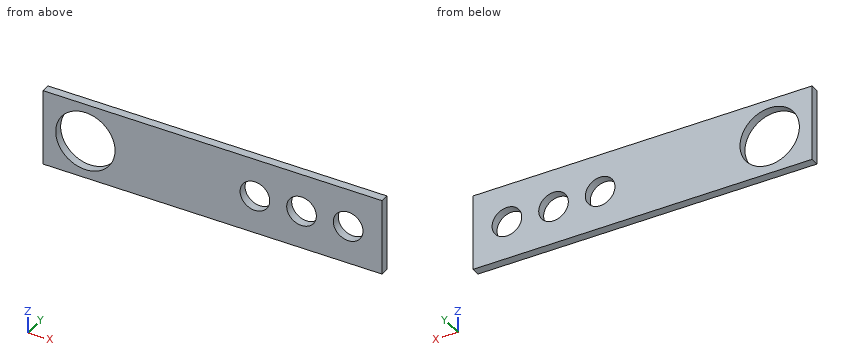
```python
from build123d import *

# Parameters (mm, degrees)
SKETCH2_W           = 40
SKETCH2_H           = 9
BOSS_EXTRUDE1_DEPTH = 1
SKETCH3_R           = 3.5
CUT_EXTRUDE1_DEPTH  = 3
SKETCH4_R           = 1.75
CUT_EXTRUDE2_DEPTH  = 3
LPATTERN1_COUNT     = 3
LPATTERN1_PITCH     = 5.5


with BuildPart() as part:
    # Sketch2 → Boss-Extrude1 (new body)
    with BuildSketch(Plane(origin=(0, 0, 0), x_dir=(1, 0, 0), z_dir=(0, 1, 0))):
        Rectangle(SKETCH2_W, SKETCH2_H)
    extrude(amount=BOSS_EXTRUDE1_DEPTH)

    # Sketch3 → Cut-Extrude1 (cut)
    with BuildSketch(Plane(origin=(0, 1, 0), x_dir=(1, 0, 0), z_dir=(0, 1, 0))):
        with Locations((-15, 0)):
            Circle(SKETCH3_R)
    extrude(amount=-CUT_EXTRUDE1_DEPTH, mode=Mode.SUBTRACT)

    # Sketch4 → Cut-Extrude2 (cut)
    with BuildSketch(Plane(origin=(0, 1, 0), x_dir=(1, 0, 0), z_dir=(0, 1, 0))):
        with Locations((5, 0)):
            Circle(SKETCH4_R)
    cut_extrude2 = extrude(amount=-CUT_EXTRUDE2_DEPTH, mode=Mode.SUBTRACT)

    # LPattern1: Cut-Extrude2 ×3
    with Locations(*[(i * LPATTERN1_PITCH, 0, 0) for i in range(1, LPATTERN1_COUNT)]):
        add(cut_extrude2, mode=Mode.SUBTRACT)


solid = part.part
```
CAD build for the part. Positions are in the model's coordinates, mm. Coordinates: 2 decimals unless noted, no trailing zeros. Write each loop counter-clockwise with the first axis right and the second up, starting at its lowest first coordinate (ties: lowest second). Pieces come first, ordered by that corner, then holes.
(1) Cut at A-A, the plane x = 5. List the corners of the cut face in (y, z), and give its area (3 significant figures).
(2) Cut at B-B, the plane z = 0. List the corners of the cut face in (x, y), and give its area (3 significant figures).
(3) Flat gauge pin, fed straight in: pin 1 (4.5 mm diameter, centred on x = 16, z = 0, fed in from -Y). Where does the tip first touch, or does it go through?
(4) Cut at D-D, the plane x = -15. List the corners of the cut face in (y, z), and give its area (3 significant figures).
(5) Cut at C-C, the plane y = 0.3. List the corners of the cut face in (x, z), and give its area (3 significant figures).
(6) Drill centre lines: probe 1 along X at (y, z) = (0.25, 0); probe 2 along Z at (x, y) = (-15, 0.8); probe 3 along Z at (x, y) = (16, 0.7). Where is each one in solid material? Low to high.
Geometry says:
1. outline: (0, -4.5) - (1, -4.5) - (1, -1.75) - (0, -1.75) - close; (0, 1.75) - (1, 1.75) - (1, 4.5) - (0, 4.5) - close
1. area: 5.50 mm2
2. outline: (-20, 0) - (-18.5, 0) - (-18.5, 1) - (-20, 1) - close; (-11.5, 0) - (3.25, 0) - (3.25, 1) - (-11.5, 1) - close; (6.75, 0) - (8.75, 0) - (8.75, 1) - (6.75, 1) - close; (12.25, 0) - (14.25, 0) - (14.25, 1) - (12.25, 1) - close; (17.75, 0) - (20, 0) - (20, 1) - (17.75, 1) - close
2. area: 22.5 mm2
3. pin 1: stops at y = 0
4. outline: (0, -4.5) - (1, -4.5) - (1, -3.5) - (0, -3.5) - close; (0, 3.5) - (1, 3.5) - (1, 4.5) - (0, 4.5) - close
4. area: 2.00 mm2
5. outline: (-20, -4.5) - (20, -4.5) - (20, 4.5) - (-20, 4.5) - close; hole circle Ø7 at (-15, 0); hole circle Ø3.5 at (5, 0); hole circle Ø3.5 at (10.5, 0); hole circle Ø3.5 at (16, 0)
5. area: 293 mm2
6. probe 1: x = -20 to -18.5, -11.5 to 3.25, 6.75 to 8.75, 12.25 to 14.25, 17.75 to 20
6. probe 2: z = -4.5 to -3.5, 3.5 to 4.5
6. probe 3: z = -4.5 to -1.75, 1.75 to 4.5
